Geometry: see drawing. Coordinates: mm, zero at the bounding-box minimum. Round coordinates to 2 decimals unless told otherwise and drop trailing zeros. Loops run counter-clockwise (first coordinate to the right, second up) from the corner with the lowest first, then second, coordinate; pieces in that order, holes last. Notation, with made-up numbers: (-3.75, -1) -> (29.25, -1) arc R6 cw to (29.25, 5) -> close; hole circle Ø5 at (58, 25.5). An arc over 180 degrees is marked (long way). Answer in a Markdown table with one row per item.
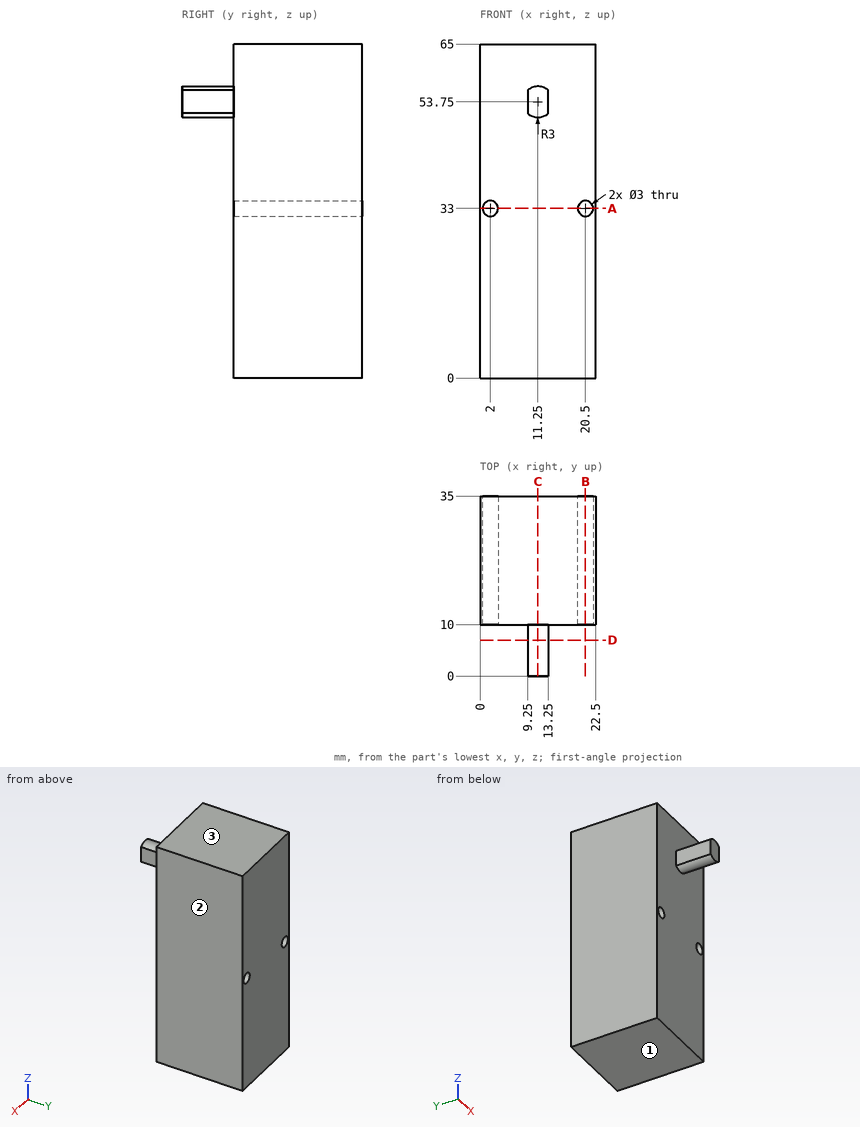
Item 1: Mould query, pull axis Z, two halves, no side actions, for the marked faces 1, 2 and 3. Classes: released by +Z, released by -Z, zero draft, split by the parting line, or undercut.
Ans:
| item | result |
|---|---|
| face 1 | released by -Z |
| face 2 | zero draft |
| face 3 | released by +Z |
Item 2: Section query B-B, the plane x = 20.5. Output: boundary loops of the cut face in (y, z).
Ans:
| item | result |
|---|---|
| outline | (10, 0) -> (35, 0) -> (35, 31.5) -> (10, 31.5) -> close; (10, 34.5) -> (35, 34.5) -> (35, 65) -> (10, 65) -> close |
Item 3: First-contact query: P1, Ø5, axis at x = 7.5, z = 42.5, coming from the -Y side; P2, Ø3, axis at y = 15, z = 32.5, coming from the -X side; P3, Ø3.5, axis at y = 3.5, z = 55, coming from the +X side; P4, Ø5, axis at y = 4, z = 54, coming from the -X side. Flat tips, straight axial feed; report the tip coordinate or a pass-through.
Ans:
| item | result |
|---|---|
| P1 | y = 10 |
| P2 | x = 0 |
| P3 | x = 13.25 |
| P4 | x = 9.25 |
Item 4: Section query A-A, the plane z = 33. Output: boundary loops of the cut face in (x, y).
Ans:
| item | result |
|---|---|
| outline | (0, 10) -> (0.5, 10) -> (0.5, 35) -> (0, 35) -> close; (3.5, 10) -> (19, 10) -> (19, 35) -> (3.5, 35) -> close; (22, 10) -> (22.5, 10) -> (22.5, 35) -> (22, 35) -> close |
Item 5: Section query C-C, the plane x = 11.25. Output: boundary loops of the cut face in (y, z), and give its area (4 significant figures).
Ans:
| item | result |
|---|---|
| outline | (0, 50.75) -> (10, 50.75) -> (10, 0) -> (35, 0) -> (35, 65) -> (10, 65) -> (10, 56.75) -> (0, 56.75) -> close |
| area | 1,685 mm2 |
Item 6: Section query D-D, the plane y = 7. Output: boundary loops of the cut face in (x, z).
Ans:
| item | result |
|---|---|
| outline | (9.25, 51.51) arc R3 ccw to (13.25, 51.51) -> (13.25, 55.99) arc R3 ccw to (9.25, 55.99) -> close |
Item 7: Ray query, L1, parallel to Z at x = 20.5, y = 24; L2, parallel to Y at x = 19, z = 22.5; L3, parallel to X at y = 3, z = 52. Return the intervals inside material, ascending.
Ans:
| item | result |
|---|---|
| L1 | 0 to 31.5, 34.5 to 65 |
| L2 | 10 to 35 |
| L3 | 9.25 to 13.25 |
